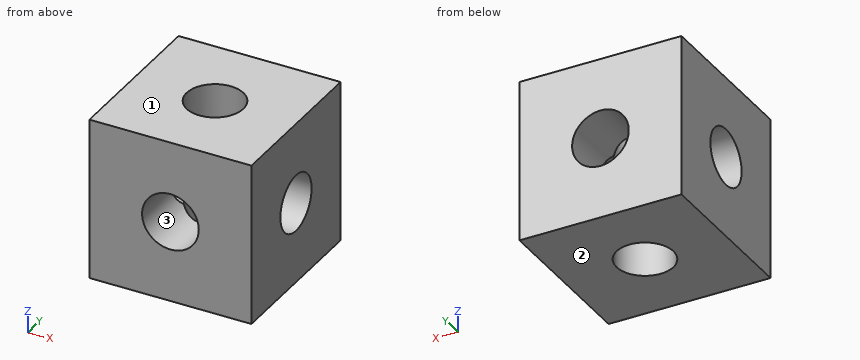
from build123d import *

# Parameters (mm, degrees)
F0_W     = 100
F0_H     = 100
F0_R     = 17.5
F1_DEPTH = 50
F2_R     = 17.5
F3_DEPTH = 100
F4_R     = 17.5
F5_DEPTH = 100


with BuildPart() as f1:
    # F0 (on Front) → F1 (new body, symmetric)
    with BuildSketch(Plane.XZ):
        Rectangle(F0_W, F0_H)
        Circle(F0_R, mode=Mode.SUBTRACT)
    extrude(amount=F1_DEPTH, both=True)

    # F2 (on face) → F3 (cut, through all)
    with BuildSketch(Plane.YZ.offset(50)):
        Circle(F2_R)
    extrude(amount=-F3_DEPTH, mode=Mode.SUBTRACT)

    # F4 (on face) → F5 (cut, through all)
    with BuildSketch(Plane.XY.offset(50)):
        Circle(F4_R)
    extrude(amount=-F5_DEPTH, mode=Mode.SUBTRACT)


solid = f1.part
For this review, take the finished solid that the model builds, in its own axes (mm). Face numbers are marked on the shaded views. Round coordinates to 2 decimals unless told otherwise and drop trailing zeros. Loops run counter-clockwise (first coordinate to the right, second up) from the corner with the lowest first, then second, coordinate; pieces in that order, holes last. Notation, with made-up numbers: (-12, 89.5) - (-4, 89.5) arc R27 cw to (-4, 117.5) - close; hole circle Ø2 at (-22, -36). An arc over 180 degrees is marked (long way). Put each result on its own line as item: value. Start each with the question number.
1. Consider section C-C on y = -31. State the section outline as (x, z) points.
2. For probe 1 along Y at (x, z) = (-29, 0), list the stretches that pass through material, from the lowest coordinate up. Write a range as [from, to].
3. Consider section A-A on z = 0. State the section outline as (x, y) points, plus the area to 4 significant figures.
4. Mouldability with a two-part tool opening along Z and no side actions: class the marked faces 1, 2 and 3 as +Z half, -Z half, draft (parallel to the pull), parting line (faces both ways), or undercut.
Result sheet:
1. outline: (-50, -50) - (50, -50) - (50, 50) - (-50, 50) - close; hole circle Ø35 at (0, 0)
2. probe 1: [-50, -17.5], [17.5, 50]
3. outline: (-50, -50) - (-17.5, -50) - (-17.5, -17.5) - (-50, -17.5) - close; (-50, 17.5) - (-17.5, 17.5) - (-17.5, 50) - (-50, 50) - close; (17.5, -50) - (50, -50) - (50, -17.5) - (17.5, -17.5) - close; (17.5, 17.5) - (50, 17.5) - (50, 50) - (17.5, 50) - close
3. area: 4,225 mm^2
4. face 1: +Z half
4. face 2: -Z half
4. face 3: undercut
